Autodesk Inventor part; units mm, degrees
ref_plane "YZ Plane" through (0, 0, 0) normal (1, 0, 0) x (0, 1, 0)
ref_plane "XZ Plane" through (0, 0, 0) normal (0, 1, 0) x (-1, 0, 0)
ref_plane "XY Plane" through (0, 0, 0) normal (0, 0, 1) x (1, 0, 0)
sketch "スケッチ1" plane through (0, 0, 0) normal (0, 0, 1) x (1, 0, 0)
  line L0 (0, 0) -> (20, 0)
  line L1 (20, 0) -> (20, 30)
  line L2 (20, 30) -> (0, 30)
  line L3 (0, 30) -> (0, 0)
  dimension "d0" = 30
  dimension "d1" = 20
extrude "押し出し1" add sketch "スケッチ1" along normal blind 2
sketch "スケッチ4" plane through (0, 0, 2) normal (0, 0, 1) x (1, 0, 0)
  line L0 (20, 30) -> (0, 30)
  line L1 (10, 30) -> (10, 0)
  line L2 (0, 0) -> (20, 0)
  point P0 (3, 5)
  point P1 (3, 25)
  point P2 (17, 5)
  point P3 (17, 25)
  dimension "d23" = 7
  dimension "d24" = 7
  dimension "d25" = 20
  dimension "d26" = 5
hole "穴3" at (3, 5, 2) at (3, 25, 2) at (17, 25, 2) at (17, 5, 2) direction (0, 0, -1) diameter 3 end through all
sketch "スケッチ5" plane through (0, 0, 2) normal (0, 0, 1) x (1, 0, 0)
  line L0 (0, 0) -> (20, 0)
  point P0 (10, 5)
  dimension "d34" = 5
hole "穴4" at (10, 5, 2) direction (0, 0, -1) diameter 3 end through all
properties part number "指支え"
The listing builds one solid part. Answer for the finished solid, in the listing's coordinates (mm). Coordinates: 2 decimals unless noted, no trailing zeros. Loops run counter-clockwise (first coordinate to the right, second up) from the corner with the lowest first, then second, coordinate; pieces in that order, holes last.
1) A flat-ended cylindrical pin translates along its axis: pin 1 Ø2.5 at (x, y) = (17, 25) entering from +Z. Find the tip coordinate at first contact, or state that the pin passes through.
2) Find the intervals of material crossed by L1, parallel to X at y = 5, z = 0.5; L2, parallel to Y at x = 17, z = 1; L3, parallel to X at y = 25, z = 1.55, in increasing order.
3) Find section B-B on x = 10. Write down the section's boundary in (y, z).
4) Find section C-C on x = 3. Write down the section's boundary in (y, z).
5) Determine the mould class of faces 1 (the face through (16.93, 26.5, 0.99)), 2 (the face through (10, 15, 0)), 3 (the face through (0, 15, 1)) for opening direction X: pulls with the +X half, pulls with the -X half, needs draft (parallel to the pull), parting line crosses it, or undercut.
6) Find section D-D on z = 1.65. Write down the section's boundary in (x, y).
7) Find section A-A on y = 5. Write down the section's boundary in (x, z), then the cut area to 3 significant figures.
Values:
1. pin 1: passes through
2. L1: x = 0 to 1.5, 4.5 to 8.5, 11.5 to 15.5, 18.5 to 20
2. L2: y = 0 to 3.5, 6.5 to 23.5, 26.5 to 30
2. L3: x = 0 to 1.5, 4.5 to 15.5, 18.5 to 20
3. outline: (0, 0) - (3.5, 0) - (3.5, 2) - (0, 2) - close; (6.5, 0) - (30, 0) - (30, 2) - (6.5, 2) - close
4. outline: (0, 0) - (3.5, 0) - (3.5, 2) - (0, 2) - close; (6.5, 0) - (23.5, 0) - (23.5, 2) - (6.5, 2) - close; (26.5, 0) - (30, 0) - (30, 2) - (26.5, 2) - close
5. face 1: undercut
5. face 2: needs draft
5. face 3: pulls with the -X half
6. outline: (0, 0) - (20, 0) - (20, 30) - (0, 30) - close; hole circle Ø3 at (3, 5); hole circle Ø3 at (3, 25); hole circle Ø3 at (10, 5); hole circle Ø3 at (17, 5); hole circle Ø3 at (17, 25)
7. outline: (0, 0) - (1.5, 0) - (1.5, 2) - (0, 2) - close; (4.5, 0) - (8.5, 0) - (8.5, 2) - (4.5, 2) - close; (11.5, 0) - (15.5, 0) - (15.5, 2) - (11.5, 2) - close; (18.5, 0) - (20, 0) - (20, 2) - (18.5, 2) - close
7. area: 22.0 mm2
